Input: part model. Units: mm. Frame: model coordinates. A direction names the side the tool comes from. Coordinates: 2 decimals unless noted, no trailing zeros. Order: outer loops, then holes, each group sorted by start corner. A loop starts at its lowest first (then second) coordinate and runs counter-clockwise, first axis right, second up. Notation, with made-up numbers: (21, 38) - (78, 38) arc R23 cw to (78, 55) - close; hole circle Ø3 at (16, 52.25). An arc over 180 degrees is marked (long way). Answer as CSV lines item,"result". Start each with the question number.
Item 1: Draft query along Z for faces 1 (the flat face through (-64.8, 1.7, -195)), 2 (the cylindrical face through (-24.9, 1, -182.5)), 3 (the flat face through (-66, 2, -126)), 4 (the flat face through (-65.2, 1.7, -55)). Return one class per face: +Z half, -Z half, draft (parallel to the pull), parting line (faces both ways), or undercut.
Item 2: Material intervals for line 1 along Z through (x, y) = (-105, 1.2); line 2 along X through (y, z) = (1.25, -185); line 3 along X through (y, z) = (4.5, -66.5), sorted ascending.
Item 3: Access query for faces 5 (the flat face through (-16, 6, -126)), 6 (the flat face through (-15, 5, -124)). Directions: +Z, -Z, +X, -X, +Y, -Y. A direction counts if a zero-diameter tool reaches every point of the face in a straight line with its end or side. Return the directions, or none.
Item 4: Section B-B (z = -65). Output: boundary loops of the cut face in (x, y).
Item 5: Section C-C (z = -179.5). Output: boundary loops of the cut face in (x, y), and give its area (3 significant figures).
Item 6: First-contact query: pin 1 (1 mm diameter, centred on x = -42.5, z = -123, fed in from -Y); pin 2 (3 mm diameter, centred on x = -103, z = -146.5, fed in from +Y). Flat tips, straight axial feed; report the tip coordinate or a pass-through.
Item 7: Section D-D (x = -86.5). Output: boundary loops of the cut face in (y, z), and give its area (3 significant figures).
Item 8: Section A-A (y = 5.5). Output: boundary loops of the cut face in (x, z), and give its area (3 significant figures).
Autodesk Inventor part; units mm, degrees
ref_plane "YZ Plane" through (0, 0, 0) normal (1, 0, 0) x (0, 1, 0)
ref_plane "XZ Plane" through (0, 0, 0) normal (0, 1, 0) x (-1, 0, 0)
ref_plane "XY Plane" through (0, 0, 0) normal (0, 0, 1) x (1, 0, 0)
sketch "Boceto1" plane through (0, 0, 0) normal (0, 1, 0) x (-1, 0, 0)
  line L0 (0, 0) -> (130, 0)
  line L1 (130, 0) -> (130, -230)
  line L2 (130, -230) -> (0, -230)
  line L3 (0, -230) -> (0, 0)
  dimension "d0" = 130
  dimension "d1" = 230
extrude "Extrusión1" add sketch "Boceto1" along normal blind 3
sketch "Boceto2" plane through (0, 3, 0) normal (0, 1, 0) x (1, 0, 0)
  line L0 (0, 230) -> (-130, 230)
  line L1 (0, 0) -> (-130, 0)
  line L2 (-130, 0) -> (-130, 230)
  line L3 (-130, 230) -> (0, 230)
  line L4 (0, 230) -> (0, 0)
  line L5 (-127, 227) -> (-127, 3)
  line L6 (-127, 3) -> (-3, 3)
  line L7 (-3, 3) -> (-3, 227)
  line L8 (-3, 227) -> (-127, 227)
  dimension "d4" = 3
extrude "Extrusión2" add sketch "Boceto2" along normal blind 60
sketch "Boceto3" plane through (-127, 3, -3) normal (1, 0, 0) x (0, 0, -1)
  line L0 (224, 0) -> (224, 60)
  line L1 (0, 60) -> (224, 60)
  line L2 (224, 60) -> (224, 59)
  line L3 (224, 59) -> (0, 59)
  line L4 (0, 59) -> (0, 60)
  point P0 (-3, -3)
  dimension "d7" = 1
extrude "Extrusión3" add sketch "Boceto3" along normal blind 10
sketch "Boceto4" plane through (-117, 3, -3) normal (1, 0, 0) x (0, 0, -1)
  line L0 (0, 59) -> (224, 59)
  line L1 (0, 60) -> (10, 60)
  line L2 (10, 60) -> (10, 59)
  line L3 (10, 59) -> (0, 59)
  line L4 (0, 59) -> (0, 60)
  line L5 (224, 60) -> (214, 60)
  line L6 (214, 60) -> (214, 59)
  line L7 (214, 59) -> (224, 59)
  line L8 (224, 59) -> (224, 60)
  point P0 (-3, -3)
  dimension "d10" = 10
  dimension "d11" = 10
extrude "Extrusión4" add sketch "Boceto4" along normal blind 115.25
sketch "Boceto5" plane through (-117, 63, -217) normal (0, 0, 1) x (1, 0, 0)
  line L0 (114, -1) -> (104, -1)
  line L1 (104, -1) -> (104, 0)
  line L2 (104, 0) -> (114, 0)
  line L3 (114, 0) -> (114, -1)
  line L4 (0, 0) -> (114, 0)
  line L5 (0, -1) -> (114, -1)
  point P0 (117, -63)
  dimension "d14" = 10
  dimension "d15" = 0
  dimension "d16" = 0
extrude "Extrusión5" add sketch "Boceto5" along normal blind 211.5
sketch "Boceto6" plane through (0, 63, 0) normal (0, 1, 0) x (1, 0, 0)
  circle A0 centre (-10, 220) radius 1.5
  circle A1 centre (-120, 220) radius 1.5
  circle A2 centre (-10, 10) radius 1.5
  circle A3 centre (-120, 10) radius 1.5
  line L0 (-130, 0) -> (0, 0)
  line L1 (0, 0) -> (0, 230)
  line L2 (-130, 230) -> (-130, 0)
  line L3 (0, 230) -> (-130, 230)
  dimension "d19" = 3
  dimension "d20" = 3
  dimension "d21" = 3
  dimension "d22" = 3
  dimension "d23" = 10
  dimension "d24" = 10
  dimension "d25" = 10
  dimension "d26" = 10
  dimension "d27" = 10
  dimension "d28" = 10
  dimension "d29" = 10
  dimension "d30" = 10
extrude "Extrusión6" cut sketch "Boceto6" against normal blind 211.5 contours A0 | A1 | A2 | A3
sketch "Boceto7" plane through (0, 0, 0) normal (0, -1, 0) x (1, 0, 0)
  circle A0 centre (-25, -205) radius 4
  circle A1 centre (-105, -205) radius 4
  circle A2 centre (-25, -25) radius 4
  circle A3 centre (-105, -25) radius 4
  line L0 (0, 0) -> (0, -230)
  line L1 (0, -230) -> (-130, -230)
  line L2 (-130, -230) -> (-130, 0)
  line L3 (-130, 0) -> (0, 0)
  dimension "d33" = 8
  dimension "d34" = 8
  dimension "d35" = 8
  dimension "d36" = 8
  dimension "d37" = 25
  dimension "d38" = 25
  dimension "d39" = 25
  dimension "d40" = 25
  dimension "d41" = 25
  dimension "d42" = 25
  dimension "d43" = 25
  dimension "d44" = 25
extrude "Extrusión7" cut sketch "Boceto7" against normal blind 10 contours A0 | A1 | A2 | A3
sketch "Boceto8" plane through (0, 0, 0) normal (0, -1, 0) x (1, 0, 0)
  line L0 (-30, -35) -> (-100, -35)
  line L1 (-100, -35) -> (-100, -45)
  line L2 (-100, -45) -> (-30, -45)
  line L3 (-30, -45) -> (-30, -35)
  line L4 (-130, 0) -> (0, 0)
  line L5 (0, 0) -> (0, -230)
  line L6 (-130, -230) -> (-130, 0)
  circle A0 centre (-35, -40) radius 2.5
  circle A1 centre (-95, -40) radius 2.5
  point P0 (-30, -40)
  dimension "d47" = 70
  dimension "d48" = 10
  dimension "d49" = 35
  dimension "d50" = 30
  dimension "d51" = 30
  dimension "d52" = 5
  dimension "d53" = 5
  dimension "d54" = 5
  dimension "d55" = 5
  dimension "d56" = 5
  dimension "d57" = 5
extrude "Extrusión8" cut sketch "Boceto8" against normal blind 10 contours A0 | A1
sketch "Boceto9" plane through (0, 0, 0) normal (0, -1, 0) x (1, 0, 0)
  line L0 (-20, -190) -> (-110, -190)
  line L1 (-110, -190) -> (-110, -60)
  line L2 (-110, -60) -> (-20, -60)
  line L3 (-20, -60) -> (-20, -190)
  line L4 (0, 0) -> (0, -230)
  line L5 (-130, -230) -> (-130, 0)
  line L6 (-130, 0) -> (0, 0)
  circle A0 centre (-25, -185) radius 2.5
  circle A1 centre (-25, -65) radius 2.5
  circle A2 centre (-105, -65) radius 2.5
  circle A3 centre (-105, -185) radius 2.5
  dimension "d60" = 90
  dimension "d61" = 130
  dimension "d62" = 20
  dimension "d63" = 20
  dimension "d64" = 60
  dimension "d65" = 5
  dimension "d66" = 5
  dimension "d67" = 5
  dimension "d68" = 5
  dimension "d69" = 5
  dimension "d70" = 5
  dimension "d71" = 5
  dimension "d72" = 5
  dimension "d73" = 5
  dimension "d74" = 5
  dimension "d75" = 5
  dimension "d76" = 5
extrude "Extrusión9" cut sketch "Boceto9" against normal blind 10 contours A0 | A1 | A2 | A3
sketch "Boceto11" plane through (0, 63, 0) normal (0, 1, 0) x (1, 0, 0)
  line L0 (-230.0178, 308.5075) -> (121.3875, 308.5075)
  line L1 (121.3875, 308.5075) -> (121.3875, -22.7652)
  line L2 (121.3875, -22.7652) -> (-230.0178, -22.7652)
  line L3 (-230.0178, -22.7652) -> (-230.0178, 308.5075)
  point P0 (0, 0)
extrude "Extrusión10" cut sketch "Boceto11" against normal blind 61
sketch "Boceto12" plane through (0, 2, 0) normal (0, 1, 0) x (1, 0, 0)
  circle A0 centre (-105, 185) radius 2.5
  circle A1 centre (-25, 65) radius 2.5
  line L0 (-105, 185) -> (-25, 185)
  line L1 (-25, 185) -> (-25, 65)
  line L2 (-25, 65) -> (-105, 65)
  line L3 (-105, 65) -> (-105, 185)
  line L4 (-158.8037, 262.2681) -> (33.433, 262.2681)
  line L5 (33.433, 262.2681) -> (33.433, -27.1386)
  line L6 (33.433, -27.1386) -> (-158.8037, -27.1386)
  line L7 (-158.8037, -27.1386) -> (-158.8037, 262.2681)
  line L8 (-15, 55) -> (-15, 195)
  line L9 (-15, 195) -> (-115, 195)
  line L10 (-115, 195) -> (-115, 55)
  line L11 (-115, 55) -> (-15, 55)
  circle A2 centre (-105, 185) radius 2.5
  circle A3 centre (-25, 185) radius 2.5
  circle A4 centre (-25, 185) radius 2.5
  circle A5 centre (-105, 65) radius 2.5
  circle A6 centre (-105, 65) radius 2.5
  circle A7 centre (-25, 65) radius 2.5
  point P0 (0, 0)
  dimension "d81" = 10
extrude "Extrusión11" cut sketch "Boceto12" against normal blind 61 contours L4 L5 L6 L7
sketch "Boceto13" plane through (-15, 2, -195) normal (0, 0, -1) x (-1, 0, 0)
  line L0 (100, 0) -> (100, -2)
  line L1 (100, -2) -> (99, -2)
  line L2 (99, -2) -> (99, 8)
  line L3 (99, 8) -> (100, 8)
  line L4 (100, 8) -> (100, -2)
  line L5 (0, -2) -> (1, -2)
  line L6 (1, -2) -> (1, 8)
  line L7 (1, 8) -> (0, 8)
  line L8 (0, 8) -> (0, -2)
  line L9 (0, 0) -> (0, -2)
  line L10 (100, 8) -> (0, 8)
  line L11 (0, 8) -> (0, 7.1109)
  line L12 (0, 7.1109) -> (100, 7.1109)
  line L13 (100, 7.1109) -> (100, 8)
  line L14 (90, 7.1109) -> (10, 7.1109)
  line L15 (10, 7.1109) -> (10, 8)
  line L16 (10, 8) -> (90, 8)
  line L17 (90, 8) -> (90, 7.1109)
  line L18 (100, 0) -> (0, 0)
  line L19 (0, 0) -> (0, 8)
  line L20 (0, 8) -> (100, 8)
  line L21 (100, 8) -> (100, 0)
  point P0 (-15, -2)
  point P1 (0, -1)
  point P2 (90, 7.5554)
  point P3 (10, 7.5554)
  point P4 (99, 0)
  point P5 (99, 7.1109)
  point P6 (10, 7.1109)
  point P7 (1, 8)
  point P8 (1, 0)
  point P9 (1, 7.1109)
  dimension "d84" = 1
  dimension "d85" = 1
  dimension "d86" = 0
  dimension "d87" = 10
  dimension "d88" = 10
  dimension "d89" = 100
  dimension "d90" = 10
  dimension "d91" = 10
extrude "Extrusión12" add sketch "Boceto13" against normal blind 140 contours L18 L2 L12 L4 | L12 L2 L3 L4 | L12 L17 L10 L2 | L18 L8 L12 L6 | L12 L8 L7 L6 | L6 L10 L15 L12
sketch "Boceto14" plane through (0, 0, 0) normal (0, -1, 0) x (1, 0, 0)
  circle A0 centre (-25, -65) radius 2.5
  circle A1 centre (-25, -65) radius 2.5
  line L0 (-25, -195) -> (-25, -55)
  circle A2 centre (-25, -185.0047) radius 2.4975
  line L1 (-105, -195) -> (-105, -55)
  circle A3 centre (-105, -185.0047) radius 2.4775
  circle A4 centre (-105, -65) radius 2.5
  circle A5 centre (-105, -65) radius 2.5
  point P0 (0, 0)
extrude "Extrusión13" cut sketch "Boceto14" against normal blind 140
Determined:
1,face 1,"-Z half"
1,face 2,"undercut"
1,face 3,"draft"
1,face 4,"+Z half"
2,line 1,"z = -195 to -187.5, -182.5 to -67.5, -62.5 to -55"
2,line 2,"x = -115 to -107.5, -102.5 to -27.5, -22.5 to -15"
2,line 3,"x = -115 to -114, -16 to -15"
3,face 5,"+Z, -Z"
3,face 6,"+Z, -Z, +X, +Y, -Y"
4,outline,"(-115, 0) - (-107.5, 0) - (-107.5, 2) - (-114, 2) - (-114, 9.11) - (-107.5, 9.11) - (-107.5, 10) - (-115, 10) - close; (-102.5, 0) - (-27.5, 0) - (-27.5, 2) - (-102.5, 2) - close; (-22.5, 0) - (-15, 0) - (-15, 10) - (-22.5, 10) - (-22.5, 9.11) - (-16, 9.11) - (-16, 2) - (-22.5, 2) - close"
5,outline,"(-115, 0) - (-15, 0) - (-15, 10) - (-25, 10) - (-25, 9.11) - (-16, 9.11) - (-16, 2) - (-114, 2) - (-114, 9.11) - (-105, 9.11) - (-105, 10) - (-115, 10) - close"
5,area,"232 mm^2"
6,pin 1,"stops at y = 0"
6,pin 2,"stops at y = 2"
7,outline,"(0, -195) - (2, -195) - (2, -55) - (0, -55) - close"
7,area,"280 mm^2"
8,outline,"(-115, -195) - (-114, -195) - (-114, -55) - (-115, -55) - close; (-16, -195) - (-15, -195) - (-15, -55) - (-16, -55) - close"
8,area,"280 mm^2"
